Autodesk Inventor part; units mm, degrees
ref_plane "作業平面1" through (514.28, 0, 15) normal (0, 0, 1) x (-1, 0, 0)
ref_plane "YZ Plane" through (0, 0, 0) normal (1, 0, 0) x (0, 1, 0)
ref_plane "XZ Plane" through (0, 0, 0) normal (0, 1, 0) x (-1, 0, 0)
sketch "スケッチ1" plane through (0, 0, 0) normal (0, 1, 0) x (-1, 0, 0)
  line L0 (-901.8, 0) -> (67, 0)
  line L1 (-417.4, -1177.3333) -> (67, 0)
  line L2 (50, -15) -> (50, 15)
  line L3 (24, 15) -> (24, -15)
  line L4 (24, -15) -> (84, -15)
  line L5 (84, 15) -> (84, -15)
  line L6 (-514.28, 15) -> (163.88, 15)
  line L7 (34, 15) -> (34, -80.2064)
  point P0 (0, 0)
  dimension "d0" = 16
ref_plane "作業平面1" through (514.28, 0, 15) normal (0, 0, 1) x (-1, 0, 0)
sketch "スケッチ2" plane through (514.28, 0, 15) normal (0, 0, 1) x (-1, 0, 0)
  line L0 (0, 0) -> (678.16, 0)
  line L1 (532.28, -16) -> (564.28, -16)
  line L2 (564.28, -16) -> (564.28, 16)
  line L3 (564.28, 16) -> (532.28, 16)
  line L4 (532.28, 16) -> (532.28, -16)
  line L5 (532.28, -16) -> (564.28, 16) construction
  line L6 (564.28, -16) -> (532.28, 16) construction
  line L7 (562.68, -14.4) -> (533.88, -14.4)
  line L8 (533.88, -14.4) -> (533.88, 14.4)
  line L9 (533.88, 14.4) -> (562.68, 14.4)
  line L10 (562.68, 14.4) -> (562.68, -14.4)
  point P0 (514.28, 0)
  point P1 (564.28, 0)
  point P2 (564.28, 0)
  point P3 (564.28, 0)
  point P4 (548.28, 0)
  point P5 (548.28, 0)
  point P6 (548.28, 0)
  dimension "d2" = 32
  dimension "d3" = 1.6
extrude "押し出し1" add sketch "スケッチ2" against normal blind 115 contours L4 L3 L2 L0 L10 L9 L8 | L0 L8 L7 L10 L2 L1 L4
sketch "スケッチ3" plane through (-50, 16, 15) normal (0, 1, 0) x (1, 0, 0)
  line L0 (467.4, 1192.3333) -> (-17, 15)
  line L1 (951.8, 15) -> (-17, 15)
  line L2 (16, 0) -> (16, 95.2064)
  point P0 (50, 15)
  point P1 (16, 95.2064)
hole "穴1" at (-34, 16, -80.2064) direction (0, -1, 0) diameter 10 end through all
properties part number "ステア棒"
Can you work these out from the model? Positions are in its coordinate system, mm. A direction names the side the tool comes from. Give positions to 0.01 mm unless a question says otherwise; leave off trailing zeros. Write each loop counter-clockwise with the first axis right and the second up, starting at its lowest first coordinate (ties: lowest second). Pieces come first, ordered by that corner, then holes. Notation, with made-up numbers: (9, -27.75) - (27, -27.75) arc R15 cw to (27, -3.75) - close; hole circle Ø2 at (48.5, -36). An arc over 180 degrees is marked (long way). Write item = value, one per line. Start each with the question number.
1. Please list where these lines run through material, in increasing order: line 1 (Y direction, x = -39, z = -53); line 2 (X direction, y = 1.5, z = -80); line 3 (Z direction, x = -34, y = 15.15).
2. On a 3-axis mill with a long thin cutter (end or side, diameter ignored), from which of +Z, -Z, +X, -X, +Y, -Y can I reach the whole of each face in a straight line? I mean faces 1 (the face through (-35.502, 15.189, -75.437)), 2 (the face through (-19.6, 0, -42)). Say none if no direction works.
3. Thinking about a two-plate mould opening in X: for faces 3 (the face through (-48.4, 0, -42)), 4 (the face through (-50, 0, -42)), 5 (the face through (-18, 0, -42)), 6 (the face through (-34, 16, -42)), which applies, released by +X, released by -X, zero draft, split by the parting line, or undercut?
4. Imagine slicing it at B-B (x = -21). Please give me the cut outline in (y, z), and give its area (3 significant figures).
5. Imagine slicing it at C-C (y = 6.5). Please give me the cut outline in (x, z), and give its area (3 significant figures).
6. Imagine slicing it at A-A (z = -8). Please give me the cut outline in (x, y).
7. Imagine slicing it at D-D (x = -34). Please give me the cut outline in (y, z), and give its area (3 significant figures).
Worked answers:
q1.line_1 = -16 to -14.4, 14.4 to 16
q1.line_2 = -50 to -48.4, -19.6 to -18
q1.line_3 = -100 to -85.21, -75.21 to 15
q2.face_1 = +Y, -Y
q2.face_2 = +Z, -Z
q3.face_3 = undercut
q3.face_4 = released by -X
q3.face_5 = released by +X
q3.face_6 = zero draft
q4.outline = (-16, -100) - (-14.4, -100) - (-14.4, 15) - (-16, 15) - close; (14.4, -100) - (16, -100) - (16, 15) - (14.4, 15) - close
q4.area = 368 mm2
q5.outline = (-50, -100) - (-48.4, -100) - (-48.4, 15) - (-50, 15) - close; (-19.6, -100) - (-18, -100) - (-18, 15) - (-19.6, 15) - close
q5.area = 368 mm2
q6.outline = (-50, -16) - (-18, -16) - (-18, 16) - (-50, 16) - close; hole (-48.4, -14.4) - (-19.6, -14.4) - (-19.6, 14.4) - (-48.4, 14.4) - close
q7.outline = (-16, -100) - (-14.4, -100) - (-14.4, -85.21) - (-16, -85.21) - close; (-16, -75.21) - (-14.4, -75.21) - (-14.4, 15) - (-16, 15) - close; (14.4, -100) - (16, -100) - (16, -85.21) - (14.4, -85.21) - close; (14.4, -75.21) - (16, -75.21) - (16, 15) - (14.4, 15) - close
q7.area = 336 mm2
